Autodesk Inventor part; units mm, degrees
ref_plane "YZ Plane" through (0, 0, 0) normal (1, 0, 0) x (0, 1, 0)
ref_plane "XZ Plane" through (0, 0, 0) normal (0, 1, 0) x (-1, 0, 0)
ref_plane "XY Plane" through (0, 0, 0) normal (0, 0, 1) x (1, 0, 0)
sketch "スケッチ1" plane through (0, 0, 0) normal (0, 0, 1) x (1, 0, 0)
  circle A0 centre (0, 0) radius 1.5
  circle A1 centre (13.5, 33.5) radius 1.25 construction
  circle A2 centre (13.5, 85.5) radius 1.25 construction
  circle A3 centre (-13.5, 85.5) radius 1.25 construction
  circle A4 centre (-13.5, 33.5) radius 1.25 construction
  circle A5 centre (0, 75) radius 1.5 construction
  circle A6 centre (0, 75) radius 13
  line L0 (16.884, 32.6064) -> (7.7349, -2.0424)
  line L1 (-7.7349, -2.0424) -> (-16.884, 32.6064)
  line L2 (-17, 33.5) -> (-17, 85.5)
  line L3 (-15.9749, 87.9749) -> (-8, 95.9497)
  line L4 (-8, 95.9497) -> (-8, 125)
  line L5 (8, 125) -> (8, 95.9497)
  line L6 (8, 95.9497) -> (15.9749, 87.9749)
  line L7 (17, 85.5) -> (17, 33.5)
  arc A7 (16.884, 32.6064) -> (17, 33.5) centre (13.5, 33.5) ccw
  arc A8 (17, 85.5) -> (15.9749, 87.9749) centre (13.5, 85.5) ccw
  arc A9 (-15.9749, 87.9749) -> (-17, 85.5) centre (-13.5, 85.5) ccw
  arc A10 (-17, 33.5) -> (-16.884, 32.6064) centre (-13.5, 33.5) ccw
  arc A11 (-7.7349, -2.0424) -> (7.7349, -2.0424) centre (0, 0) ccw
  line L8 (0, 0) -> (0, 152.1421) construction
  arc A12 (8, 125) -> (-8, 125) centre (0, 125) ccw
  point P0 (0, 113)
  dimension "d2" = 3
  dimension "d3" = 26
  dimension "d4" = 3.5
  dimension "d5" = 8
  dimension "d6" = 125
  dimension "d7" = 16
  dimension "d8" = 45
  dimension "d9" = 45
  dimension "d10" = 38
extrude "押し出し1" add sketch "スケッチ1" along normal blind 2
hole "穴2" at (0, 125, 0) direction (0, 0, 1) diameter 8 end through all
hole "穴3" at (0, 113, 0) direction (0, 0, 1) diameter 6 end through all
fillet "フィレット1" radius 6.5 2 edges at (-8, 95.9497, 1) (8, 95.9497, 1)
sketch "スケッチ2" plane through (0, 0, 2) normal (0, 0, 1) x (1, 0, 0)
  arc A0 (17, 85.5) -> (15.9749, 87.9749) centre (13.5, 85.5) ccw construction
  arc A1 (-15.9749, 87.9749) -> (-17, 85.5) centre (-13.5, 85.5) ccw construction
  arc A2 (-17, 33.5) -> (-16.884, 32.6064) centre (-13.5, 33.5) ccw construction
  arc A3 (16.884, 32.6064) -> (17, 33.5) centre (13.5, 33.5) ccw construction
  point P0 (0, 0)
hole "穴4" at (13.5, 85.5, 2) at (-13.5, 85.5, 2) at (-13.5, 33.5, 2) at (13.5, 33.5, 2) direction (0, 0, -1) diameter 2.6 end through all countersink diameter 5.5 countersink angle 90
properties part number "UPPER_LEG_BASE"
Geometry: final body of the model. Coordinates: model frame, mm. Give positions to 0.01 mm unless a question says otherwise; leave off trailing zeros. Order: outer loops, then holes, each group sorted by start corner. A loop starts at its lowest first (then second) coordinate and runs counter-clockwise, first axis right, second up. Notation, with made-up numbers: (8.5, -4.5) -> (57.5, -4.5) arc R18 ccw to (57.5, 17.5) -> close; hole circle Ø3 at (24.25, -17). An arc over 180 degrees is marked (long way). Write each question's results on one line, items separated by ' | '. Start each with the question number.
1) Section B-B (z = 1.15). Count the separate pieces of the cut face and the enclosed holes in it, then the cut area to 3 significant figures.
2) Section A-A (y = 75). Return loops of the section in (x, z).
3) Line query: line 1 (X direction, y = 33.5, z = 0.2); line 2 (X direction, y = 85.5, z = 0.3); line 3 (Y direction, x = 1, z = 0.2). Output: solid intervals per line, ascending. Write a range as from..to.
4) Draft query along Y for faces 1 (the flat face through (0, 48, 0)), 2 (the cylindrical face through (13.44, 34.8, 0.27)), 3 (the cylindrical face through (0, 133, 1)). Return one class per face: pulls with the +Y half, pulls with the -Y half, needs draft (parallel to the pull), parting line crosses it, or undercut.
5) First-contact query: pin 1 (2.5 mm diameter, centred on x = 0, y = 0, fed in from -Z); pin 2 (1 mm diameter, centred on y = 115, z = 1, fed in from -X). Flat tips, straight axial feed; report the tip coordinate or a pass-through.
6) Section D-D (y = 113). Return loops of the section in (x, z), then the cut area to 3 significant figures.
7) Section C-C (x = 0). Return loops of the section in (y, z), then the cut area to 3 significant figures.
Calculated:
1) separate pieces: 1 | enclosed holes: 8 | area: 2,900 mm2
2) outline: (-17, 0) -> (-13, 0) -> (-13, 2) -> (-17, 2) -> close; (13, 0) -> (17, 0) -> (17, 2) -> (13, 2) -> close
3) line 1: -17..-14.8, -12.2..12.2, 14.8..17 | line 2: -17..-14.8, -12.2..-7.66, 7.66..12.2, 14.8..17 | line 3: -7.94..-1.12, 1.12..62.04, 87.96..110.17, 115.83..121.13, 128.87..132.94
4) face 1: needs draft | face 2: undercut | face 3: pulls with the +Y half
5) pin 1: through | pin 2: x = -8
6) outline: (-8, 0) -> (-3, 0) -> (-3, 2) -> (-8, 2) -> close; (3, 0) -> (8, 0) -> (8, 2) -> (3, 2) -> close | area: 20.0 mm2
7) outline: (-8, 0) -> (-1.5, 0) -> (-1.5, 2) -> (-8, 2) -> close; (1.5, 0) -> (62, 0) -> (62, 2) -> (1.5, 2) -> close; (88, 0) -> (110, 0) -> (110, 2) -> (88, 2) -> close; (116, 0) -> (121, 0) -> (121, 2) -> (116, 2) -> close; (129, 0) -> (133, 0) -> (133, 2) -> (129, 2) -> close | area: 196 mm2
